Could you check a few things on this model? Use its own coordinates, in mm. Face numbers are marked on the shaded views. A direction names the side the tool comes from. Coordinates: 2 decimals unless noted, no trailing zeros. Loops run counter-clockwise (first coordinate to the right, second up) from the corner with the lowest first, then second, coordinate; pieces in that order, holes last. Notation, with made-up numbers: (15.5, 53.25) - (29.5, 53.25) arc R34 cw to (29.5, 90.25) - close; hole circle Ø6 at (15.25, -1). An arc over 180 degrees is marked (long way). Use CSV: the item, a comma, the result in double quotes.
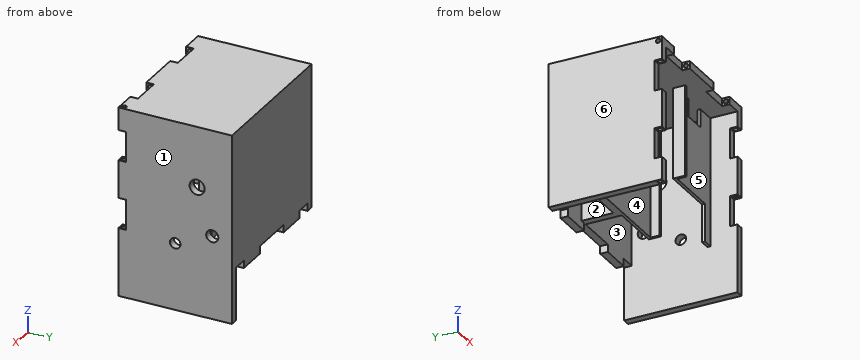
from build123d import *

# Parameters (mm, degrees)
VOLUME_BOITIER_DEPTH     = 90
ESQUISSE2_W              = 100
ESQUISSE2_H              = 75
FACE_INF_RIEURE_DEPTH    = 5
ESQUISSE3_W              = 5
ESQUISSE3_H              = 75
FACE_PILE_DEPTH          = 30
ESQUISSE7_W              = 5
ESQUISSE7_H              = 20
ESQUISSE7_W_2            = 20
ESQUISSE7_H_2            = 5
ENL_V_MAT_EXTRU_2_DEPTH  = 5
ESQUISSE8_R              = 1.5
ENL_V_MAT_EXTRU_3_DEPTH  = 93
ESQUISSE9_R              = 1.5
ENL_V_MAT_EXTRU_4_DEPTH  = 88
ESQUISSE10_R             = 1.5
ENL_V_MAT_EXTRU_5_DEPTH  = 87
ENL_V_MAT_EXTRU_6_REACH  = 159.003
ESQUISSE11_R             = 3.5
ESQUISSE14_W             = 10
ESQUISSE14_H             = 5
ESQUISSE14_W_2           = 30
ENL_V_MAT_EXTRU_8_DEPTH  = 5
BOSS_EXTRU_7_DEPTH       = 85
ENL_V_MAT_EXTRU_10_REACH = 151.245
ESQUISSE15_W             = 15
ESQUISSE15_H             = 12
ENL_V_MAT_EXTRU_11_REACH = 159.003
ESQUISSE16_R             = 4
ESQUISSE16_R_2           = 5
ENL_V_MAT_EXTRU_12_DEPTH = 25


with BuildPart() as part:
    # Esquisse1 → volume boitier (new body)
    with BuildSketch(Plane.XY):
        Polygon((0, 75), (0, 0), (5, 0), (5, 70), (95, 70), (95, 0), (100, 0), (100, 75), align=None)
    extrude(amount=VOLUME_BOITIER_DEPTH)

    # Esquisse2 → face inférieure (add)
    with BuildSketch(Plane.XY.offset(90)):
        with Locations((50, 37.5)):
            Rectangle(ESQUISSE2_W, ESQUISSE2_H)
    extrude(amount=FACE_INF_RIEURE_DEPTH)

    # Esquisse3 → face pile (add)
    with BuildSketch(Plane(origin=(0, 0, 0), x_dir=(-1, 0, 0), z_dir=(0, 0, -1))):
        with Locations((-97.5, 37.5)):
            Rectangle(ESQUISSE3_W, ESQUISSE3_H)
    extrude(amount=FACE_PILE_DEPTH)

    # Esquisse7 → Enlèv. mat.-Extru.2 (cut)
    with BuildSketch(Plane.XZ):
        with Locations((2.5, 25)):
            Rectangle(ESQUISSE7_W, ESQUISSE7_H)
        with Locations((2.5, 70)):
            Rectangle(ESQUISSE7_W, ESQUISSE7_H)
        with Locations((25, 92.5)):
            Rectangle(ESQUISSE7_W_2, ESQUISSE7_H_2)
        with Locations((75, 92.5)):
            Rectangle(ESQUISSE7_W_2, ESQUISSE7_H_2)
        with Locations((97.5, 70)):
            Rectangle(ESQUISSE7_W, ESQUISSE7_H)
        with Locations((97.5, 25)):
            Rectangle(ESQUISSE7_W, ESQUISSE7_H)
    extrude(amount=-ENL_V_MAT_EXTRU_2_DEPTH, mode=Mode.SUBTRACT)

    # Esquisse8 → Enlèv. mat.-Extru.3 (cut)
    with BuildSketch(Plane.ZY):
        with Locations((92.5, 2.5)):
            Circle(ESQUISSE8_R)
    extrude(amount=-ENL_V_MAT_EXTRU_3_DEPTH, mode=Mode.SUBTRACT)

    # Esquisse9 → Enlèv. mat.-Extru.4 (cut)
    with BuildSketch(Plane(origin=(0, 0, 0), x_dir=(-1, 0, 0), z_dir=(0, 0, -1))):
        with Locations((-2.5, 2.5)):
            Circle(ESQUISSE9_R)
    extrude(amount=-ENL_V_MAT_EXTRU_4_DEPTH, mode=Mode.SUBTRACT)

    # Esquisse10 → Enlèv. mat.-Extru.5 (cut)
    with BuildSketch(Plane.XY.offset(95)):
        with Locations(Location((97.5, 2.5, 0), (0, 0, 180))):
            Circle(ESQUISSE10_R)
    extrude(amount=-ENL_V_MAT_EXTRU_5_DEPTH, mode=Mode.SUBTRACT)

    # Esquisse11 → Enlèv. mat.-Extru.6 (cut, up to next)
    with BuildSketch(Plane(origin=(100, 0, 0), x_dir=(0, 0, -1), z_dir=(1, 0, 0)), mode=Mode.PRIVATE) as enl_v_mat_extru_6_sk1:
        with Locations((-14.229443479, 37.5)):
            Circle(ESQUISSE11_R)
    enl_v_mat_extru_6_tool1 = extrude(enl_v_mat_extru_6_sk1.sketch, amount=-ENL_V_MAT_EXTRU_6_REACH, mode=Mode.PRIVATE) & part.part
    add(enl_v_mat_extru_6_tool1.solids().sort_by_distance((100, 37.5, 14.229443))[0], mode=Mode.SUBTRACT)

    # Esquisse14 → Enlèv. mat.-Extru.8 (cut)
    with BuildSketch(Plane(origin=(0, 0, 0), x_dir=(-1, 0, 0), z_dir=(0, 0, -1))):
        with Locations((-90, 72.5)):
            Rectangle(ESQUISSE14_W, ESQUISSE14_H)
        with Locations((-50, 72.5)):
            Rectangle(ESQUISSE14_W_2, ESQUISSE14_H)
        with Locations((-10, 72.5)):
            Rectangle(ESQUISSE14_W, ESQUISSE14_H)
    extrude(amount=-ENL_V_MAT_EXTRU_8_DEPTH, mode=Mode.SUBTRACT)

    # Esquisse12 → Boss.-Extru.7 (add)
    with BuildSketch(Plane(origin=(0, 0, 90), x_dir=(-1, 0, 0), z_dir=(0, 0, -1))):
        Polygon((-37, 46), (-70.75, 46), (-70.75, 38), (-69.25, 38), (-69.25, 44), (-5, 44), (-5, 49), (-32, 49), (-32, 70), (-37, 70), align=None)
        Polygon((-52, 16.786904399), (-52, 12), (-53.5, 12), (-53.5, 18), (-95, 18), (-95, 20), (-52, 20), align=None)
    extrude(amount=BOSS_EXTRU_7_DEPTH)

    # Esquisse15 → Enlèv. mat.-Extru.10 (cut, up to next)
    with BuildSketch(Plane.XZ.offset(-18), mode=Mode.PRIVATE) as enl_v_mat_extru_10_sk1:
        with Locations((75, 84)):
            Rectangle(ESQUISSE15_W, ESQUISSE15_H)
    enl_v_mat_extru_10_tool1 = extrude(enl_v_mat_extru_10_sk1.sketch, amount=-ENL_V_MAT_EXTRU_10_REACH, mode=Mode.PRIVATE) & part.part
    add(enl_v_mat_extru_10_tool1.solids().sort_by_distance((75, 18, 84))[0], mode=Mode.SUBTRACT)

    # Esquisse16 → Enlèv. mat.-Extru.11 (cut, up to next)
    with BuildSketch(Plane(origin=(100, 0, 0), x_dir=(0, 0, -1), z_dir=(1, 0, 0)), mode=Mode.PRIVATE) as enl_v_mat_extru_11_sk1:
        with Locations((-25, 62)):
            Circle(ESQUISSE16_R)
    enl_v_mat_extru_11_tool1 = extrude(enl_v_mat_extru_11_sk1.sketch, amount=-ENL_V_MAT_EXTRU_11_REACH, mode=Mode.PRIVATE) & part.part
    # Esquisse16 → Enlèv. mat.-Extru.11 (cut, up to next)
    with BuildSketch(Plane(origin=(100, 0, 0), x_dir=(0, 0, -1), z_dir=(1, 0, 0)), mode=Mode.PRIVATE) as enl_v_mat_extru_11_sk2:
        with Locations((-55, 52)):
            Circle(ESQUISSE16_R_2)
    enl_v_mat_extru_11_tool2 = extrude(enl_v_mat_extru_11_sk2.sketch, amount=-ENL_V_MAT_EXTRU_11_REACH, mode=Mode.PRIVATE) & part.part
    add(enl_v_mat_extru_11_tool1.solids().sort_by_distance((100, 62, 25))[0], mode=Mode.SUBTRACT)
    add(enl_v_mat_extru_11_tool2.solids().sort_by_distance((100, 52, 55))[0], mode=Mode.SUBTRACT)

    # Esquisse17 → Enlèv. mat.-Extru.12 (cut)
    with BuildSketch(Plane(origin=(0, 0, 5), x_dir=(-1, 0, 0), z_dir=(0, 0, -1))):
        Polygon((-88.283089538, 20), (-52, 20), (-52, 12), (-53.5, 12), (-53.5, 18), (-88.283089538, 18), align=None)
    extrude(amount=-ENL_V_MAT_EXTRU_12_DEPTH, mode=Mode.SUBTRACT)


solid = part.part
(1) Suppose I cut it at C-C (y = 62). Write out the boundary of the cut face in (x, z), plus the area to 4 significant figures.
Computed:
outline,"(0, 0) - (5, 0) - (5, 90) - (32, 90) - (32, 5) - (37, 5) - (37, 90) - (95, 90) - (95, 29) - (100, 29) - (100, 95) - (0, 95) - close; (95, -30) - (100, -30) - (100, 21) - (95, 21) - close"
area,"1,935 mm²"
(2) Will these pins go through, and if not, where does the flat tip stop? pin 1 (4 mm diameter, centred on x = 96.5, z = 20.5, fed in from -Y); pin 2 (1.5 mm diameter, centred on x = 11.5, y = 71.5, fed in from -Z); pin 3 (19.5 mm diameter, centred on x = 51, z = 39.5, fed in from -Y).
Computed:
pin 1,"stops at y = 5"
pin 2,"stops at z = 5"
pin 3,"stops at y = 12"
(3) Suppose I cut it at A-A (x = 2.5). Write out the boundary of the cut face in (y, z), plus the area to 3 significant figures.
Computed:
outline,"(0, 0) - (1, 0) - (1, 15) - (0, 15) - close; (0, 35) - (1, 35) - (1, 60) - (0, 60) - close; (0, 80) - (1, 80) - (1, 88) - (4, 88) - (4, 80) - (5, 80) - (5, 60) - (4, 60) - (4, 35) - (5, 35) - (5, 15) - (4, 15) - (4, 0) - (75, 0) - (75, 95) - (0, 95) - close; hole circle Ø3 at (2.5, 92.5)"
area,"6,770 mm²"
(4) Thinking about a two-plate mould opening in Y: for the marked faces 3, 4, 5 and 6, which applies, +Y half, -Y half, draft (parallel to the pull), parting line (faces both ways), or undercut?
Computed:
face 3,"undercut"
face 4,"undercut"
face 5,"-Y half"
face 6,"draft"
(5) Please list where these lines run through material, in increasing order: line 1 (Y direction, x = 97.5, z = 13.75); line 2 (X direction, y = 65.5, z = 11); line 3 (X direction, y = 40, z = 52).
Computed:
line 1,"y = 0 to 1, 4 to 34.03, 40.97 to 75"
line 2,"x = 0 to 5, 32 to 37, 95 to 100"
line 3,"x = 0 to 5, 69.25 to 70.75, 95 to 100"
(6) Suppose I cut it at B-B (z = 25). Write out the boundary of the cut face in (x, y), plus the area to 3 significant figures.
Computed:
outline,"(0, 5) - (5, 5) - (5, 44) - (69.25, 44) - (69.25, 38) - (70.75, 38) - (70.75, 46) - (37, 46) - (37, 70) - (95, 70) - (95, 66) - (100, 66) - (100, 75) - (0, 75) - close; (88.28, 18) - (95, 18) - (95, 5) - (100, 5) - (100, 58) - (95, 58) - (95, 20) - (88.28, 20) - close; hole (5, 49) - (32, 49) - (32, 70) - (5, 70) - close"
area,"1,460 mm²"
(7) Suppose I cut it at D-D (z = 40). Write out the boundary of the cut face in (x, y), plus the area to 3 significant figures.
Computed:
outline,"(0, 0) - (5, 0) - (5, 44) - (69.25, 44) - (69.25, 38) - (70.75, 38) - (70.75, 46) - (37, 46) - (37, 70) - (95, 70) - (95, 20) - (52, 20) - (52, 12) - (53.5, 12) - (53.5, 18) - (95, 18) - (95, 0) - (100, 0) - (100, 75) - (0, 75) - close; hole circle Ø3 at (2.5, 2.5); hole (5, 49) - (32, 49) - (32, 70) - (5, 70) - close; hole circle Ø3 at (97.5, 2.5)"
area,"1,620 mm²"
(8) Which directions (+Z, -Z, +X, -X, +Y, -Y) give clear straight access to the entire face, cutting with the end or side of a thin tool? Please do the marked faces 1 and 2.
Computed:
face 1,"+Z, -Z, +X, +Y, -Y"
face 2,"-Z"
